Could you check a few things on this model? Use its own coordinates, in mm. Face numbers are marked on the shaded views. Round coordinates to 2 decimals unless told otherwise and drop trailing zeros. Write each loop counter-clockwise with the first axis right and the second up, starting at its lowest first coordinate (ties: lowest second). Pieces come first, ordered by that corner, then holes. Notation, with made-up numbers: (66, -11) - (76, -11) arc R13 ccw to (76, -1) - close; hole circle Ø5 at (60, 11). An arc over 180 degrees is marked (long way). Put each result on its own line as item: value.
from build123d import *

# Parameters (mm, degrees)
SKETCH1_W           = 120
SKETCH1_H           = 78
BOSS_EXTRUDE1_DEPTH = 24
FILLET1_R           = 15
FILLET2_R           = 1
BOSS_EXTRUDE2_DEPTH = 8
SKETCH2_3_R         = 4
CUT_EXTRUDE1_DEPTH  = 8


with BuildPart() as part:
    # Sketch1 → Boss-Extrude1 (new body)
    with BuildSketch(Plane.XY):
        Rectangle(SKETCH1_W, SKETCH1_H)
    extrude(amount=BOSS_EXTRUDE1_DEPTH)

    # Fillet1
    fillet1_edges = [part.edges().sort_by_distance(p)[0] for p in [
        (-60, 0, 24),
    ]]
    fillet(fillet1_edges, radius=FILLET1_R)

    # Fillet2
    fillet2_edges = [part.edges().sort_by_distance(p)[0] for p in [
        (7.5, -39, 24),
        (-60, -39, 4.5),
        (-55.606601718, -39, 19.606601718),
        (-60, 39, 4.5),
        (-55.606601718, 39, 19.606601718),
        (60, 0, 24),
        (0, -39, 0),
        (-60, 0, 0),
        (0, 39, 0),
        (60, 0, 0),
        (60, -39, 12),
        (60, 39, 12),
        (7.5, 39, 24),
    ]]
    fillet(fillet2_edges, radius=FILLET2_R)

    # Sketch2 → Boss-Extrude2 (add)
    with BuildSketch(Plane(origin=(0, -39, 0), x_dir=(-1, 0, 0), z_dir=(0, -1, 0))):
        with BuildLine():
            Line((16, -19.249615362), (16, -19.872983346))
            ThreePointArc((16, -19.872983346), (15, -12), (14, -19.872983346))
            Line((14, -19.872983346), (14, -19.249615362))
            ThreePointArc((14, -19.249615362), (15, -12.6), (16, -19.249615362))
        make_face()
        with BuildLine():
            ThreePointArc((-4, -19.872983346), (-5, -12), (-6, -19.872983346))
            Line((-6, -19.872983346), (-6, -19.249615362))
            ThreePointArc((-6, -19.249615362), (-5, -12.6), (-4, -19.249615362))
            Line((-4, -19.249615362), (-4, -19.872983346))
        make_face()
        with BuildLine():
            ThreePointArc((-24, -19.872983346), (-25, -12), (-26, -19.872983346))
            Line((-26, -19.872983346), (-26, -19.249615362))
            ThreePointArc((-26, -19.249615362), (-25, -12.6), (-24, -19.249615362))
            Line((-24, -19.249615362), (-24, -19.872983346))
        make_face()
        with BuildLine():
            ThreePointArc((-44, -19.872983346), (-45, -12), (-46, -19.872983346))
            Line((-46, -19.872983346), (-46, -19.249615362))
            ThreePointArc((-46, -19.249615362), (-45, -12.6), (-44, -19.249615362))
            Line((-44, -19.249615362), (-44, -19.872983346))
        make_face()
    extrude(amount=BOSS_EXTRUDE2_DEPTH)

    # Sketch2<3> → Cut-Extrude1 (cut)
    with BuildSketch(Plane(origin=(0, -39, 0), x_dir=(-1, 0, 0), z_dir=(0, -1, 0))):
        with Locations((35, -16)):
            Circle(SKETCH2_3_R)
    extrude(amount=-CUT_EXTRUDE1_DEPTH, mode=Mode.SUBTRACT)


solid = part.part
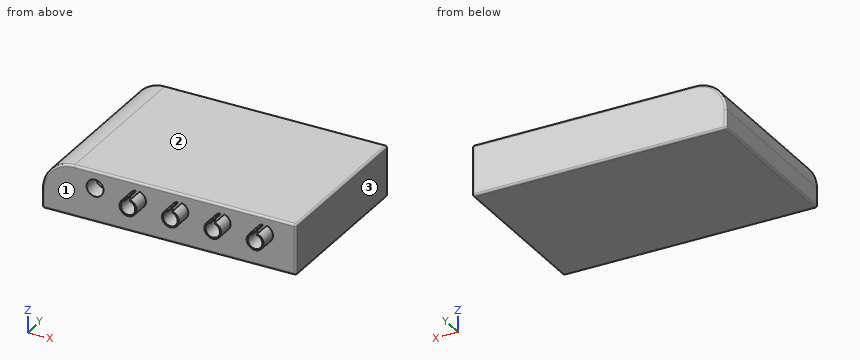
(1) Imagine slicing it at A-A, the plane y = 32.5. List the corners of the cut face in (x, z) for me, then the cut area to 3 significant figures.
Values found:
outline: (-60, 1) arc R1 ccw to (-59, 0) - (59, 0) arc R1 ccw to (60, 1) - (60, 23) arc R1 ccw to (59, 24) - (-45, 24) arc R15 ccw to (-60, 9) - close
area: 2,830 mm^2
(2) Imagine slicing it at B-B, the plane x = -35. List the corners of the cut face in (y, z) for me, then the cut area to 3 significant figures.
Values found:
outline: (-39, 1) arc R1 ccw to (-38, 0) - (38, 0) arc R1 ccw to (39, 1) - (39, 23) arc R1 ccw to (38, 24) - (-38, 24) arc R1 ccw to (-39, 23) - (-39, 20) - (-31, 20) - (-31, 12) - (-39, 12) - close
area: 1,810 mm^2
(3) If we mould it in two halves opening along X, with no side actions, what happens to the marked faces 1, 2 and 3? For each: pulls with the +X half, pulls with the -X half, needs draft (parallel to the pull), parting line crosses it, or undercut.
Values found:
face 1: undercut
face 2: needs draft
face 3: pulls with the +X half
(4) I'm going to push flat-ended pins straight in: pin 1 (9 mm diameter, centred on x = -33, z = 17, fed in from -Y); pin 2 (3 mm diameter, centred on y = -14.5, z = 21, fed in from -X); pin 3 (1 mm diameter, centred on y = -4, z = 13.5, fed in from -X). Where does each tip first touch, or does it pass through?
Values found:
pin 1: stops at y = -39
pin 2: stops at x = -55.71
pin 3: stops at x = -59.46
(5) Please list where these lines run through material, in increasing order: probe 1 along Z at (x, y) = (-35, -36.75); probe 2 along Z at (x, y) = (-15, -45); probe 3 along Y at (x, z) = (29, 10.25). Write a range as from..to.
Values found:
probe 1: z = 0..12, 20..24
probe 2: z = 12..12.6
probe 3: y = -39..39
